Answer from the drawing. Dimensions are ordinates in mm from the lowest x, y and z of the part. A direction names the side the tool comes from. Give positions to 0.01 mm unless a question says otherwise; leave off trailing zeros. Loops run counter-clockwise (first coordinate to the right, second up) from the corner with the lowest first, then second, coordinate; pieces in that order, holes last. Notation, with made-up numbers: (-21.5, -40) - (-16.5, -40) arc R12 cw to (-16.5, -26) - close; hole circle Ø9 at (54.25, 60). An arc over 180 degrees is marked (long way). Write each question's results on one line, items separated by ' | '. Start each with the question number.
Q1. For the marked faces 5 and 6, determine the directions among +Z, -Z, +X, -X, +Y, -Y from which every point of the face is accessible in a straight line to the end or side of a thin tool.
Q2. Given pin 1 (1.5 mm diameter, centred on x = 22.5, y = 4.5, fed in from +Z), flat-ended and moving along its own axis, determine where the tip first touches the part or whether it passes through.
Q3. Determine the mould class of the marked faces 1, 2, 3 and 4 for opening direction Y: +Y half, -Y half, draft (parallel to the pull), parting line (faces both ways), or undercut.
Q4. The part is cut by section A-A, the plane x = 8. Write down the section's boundary in (y, z).
Q5. The part is cut by section B-B, the plane z = 5. Write down the section's boundary in (x, y).
Q6. Find the intervals of material crossed by line 1 (Y direction, x = 20.5, z = 1.75); line 2 (X direction, y = 5.25, z = 0.75), in increasing order. Write a range as from..to.
Q7. The part is cut by section C-C, the plane y = 6. Write down the section's boundary in (x, z), plus the area to 3 significant figures.
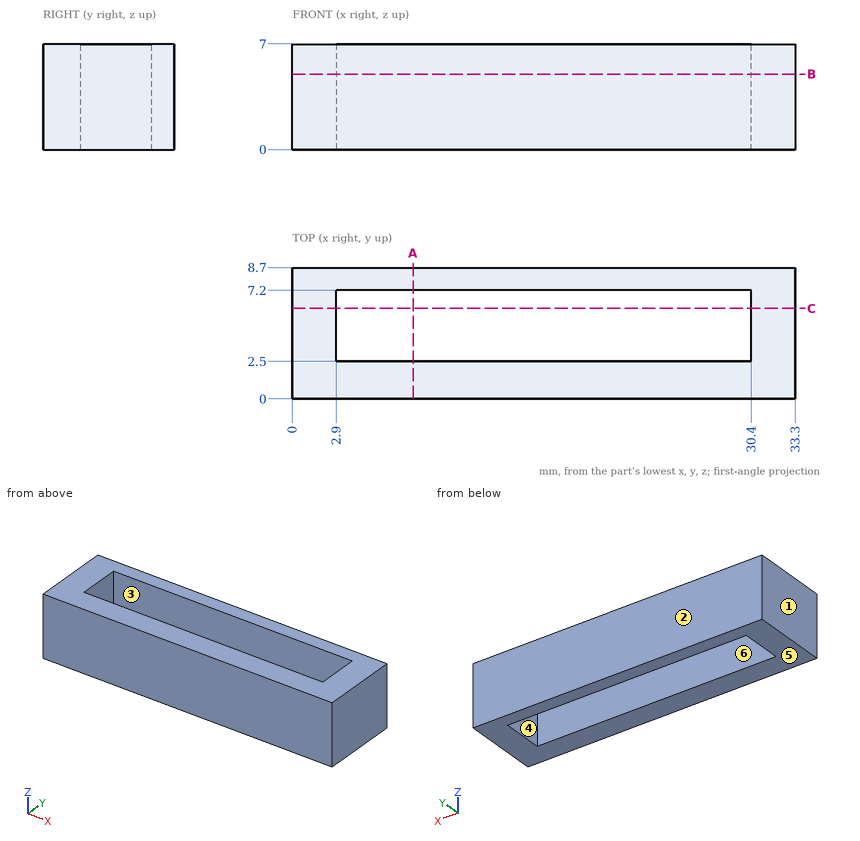
Check sheet entries:
1) face 5: -Z, +X, -X, +Y, -Y | face 6: +Z, -Z
2) pin 1: passes through
3) face 1: draft | face 2: +Y half | face 3: undercut | face 4: undercut
4) outline: (0, 0) - (2.5, 0) - (2.5, 7) - (0, 7) - close; (7.2, 0) - (8.7, 0) - (8.7, 7) - (7.2, 7) - close
5) outline: (0, 0) - (33.3, 0) - (33.3, 8.7) - (0, 8.7) - close; hole (2.9, 2.5) - (30.4, 2.5) - (30.4, 7.2) - (2.9, 7.2) - close
6) line 1: y = 0..2.5, 7.2..8.7 | line 2: x = 0..2.9, 30.4..33.3
7) outline: (0, 0) - (2.9, 0) - (2.9, 7) - (0, 7) - close; (30.4, 0) - (33.3, 0) - (33.3, 7) - (30.4, 7) - close | area: 40.6 mm^2
